Autodesk Inventor part; units mm, degrees
ref_plane "YZ Plane" through (0, 0, 0) normal (1, 0, 0) x (0, 1, 0)
ref_plane "XZ Plane" through (0, 0, 0) normal (0, 1, 0) x (-1, 0, 0)
ref_plane "XY Plane" through (0, 0, 0) normal (0, 0, 1) x (1, 0, 0)
sketch "Sketch1" plane through (0, 0, 0) normal (1, 0, 0) x (0, 1, 0)
  line L0 (0, 0) -> (25.4, 0)
  line L1 (0, 0) -> (0, -25.4)
  line L2 (25.4, -6.35) -> (6.35, -6.35)
  line L3 (6.35, -6.35) -> (6.35, -25.4)
  line L4 (6.35, -25.4) -> (0, -25.4)
  line L5 (25.4, 0) -> (25.4, -6.35)
  dimension "d0" = 25.4
  dimension "d1" = 25.4
  dimension "d2" = 6.35
extrude "Extrusion1" add sketch "Sketch1" along normal mid plane 120
sketch "Sketch2" plane through (-60, 6.35, -6.35) normal (0, 1, 0) x (1, 0, 0)
  circle A0 centre (10, 9.525) radius 4.1
  line L0 (0, 0) -> (0, 19.05) construction
  line L1 (0, 19.05) -> (120, 19.05) construction
  circle A1 centre (30, 9.525) radius 4.1
  circle A2 centre (50, 9.525) radius 4.1
  circle A3 centre (70, 9.525) radius 4.1
  circle A4 centre (90, 9.525) radius 4.1
  circle A5 centre (110, 9.525) radius 4.1
  point P0 (60, -6.35)
  point P1 (0, 9.525)
  point P2 (0, 9.525)
  dimension "d5" = 8.2
  dimension "d6" = 10
  dimension "d9" = 20
hole "Hole1" at (50, 6.35, -15.875) at (30, 6.35, -15.875) at (10, 6.35, -15.875) at (-10, 6.35, -15.875) at (-30, 6.35, -15.875) at (-50, 6.35, -15.875) direction (0, -1, 0) diameter 8.2 end through all countersink diameter 14 countersink angle 90
sketch "Sketch3" plane through (60, 25.4, -6.35) normal (0, 0, -1) x (-1, 0, 0)
  circle A0 centre (10, -9.525) radius 4
  line L0 (0, -19.05) -> (0, 0) construction
  line L1 (120, 0) -> (0, 0) construction
  circle A1 centre (30, -9.525) radius 4
  circle A2 centre (50, -9.525) radius 4
  circle A3 centre (70, -9.525) radius 4
  circle A4 centre (90, -9.525) radius 4
  circle A5 centre (110, -9.525) radius 4
  point P0 (60, -25.4)
  point P1 (0, -9.525)
  dimension "d21" = 8
  dimension "d22" = 10
  dimension "d25" = 20
hole "Hole2" at (50, 15.875, -6.35) at (30, 15.875, -6.35) at (10, 15.875, -6.35) at (-10, 15.875, -6.35) at (-30, 15.875, -6.35) at (-50, 15.875, -6.35) direction (0, 0, 1) diameter 8.2 end through all countersink diameter 14 countersink angle 90
properties part number "MotorMountingBracket"
Source: CAD feature listing. Evaluate the final solid. Frame: model axes, mm. A direction names the side the tool comes from. Coordinates: 2 decimals unless noted, no trailing zeros. Order: outer loops, then holes, each group sorted by start corner. A loop starts at its lowest first (then second) coordinate and runs counter-clockwise, first axis right, second up. Notation, with made-up numbers: M -13.5,16 L -0.5,16 A10 cw -0.5,30 Z; hole C 85.5,1 d8. An arc over 180 degrees is marked long. Write each question's results on one line, items separated by ' | '. Start each with the question number.
1) Section query A-A (x = 10). Return the cut outline in (y, z) (3 decimals), plus the area to 3 significant figures.
2) Contact query for flat-ended pins moving along their axis: pin 1 Ø13 at (x, z) = (30, -15.875) entering from +Y; pin 2 Ø13 at (x, y) = (-30, 15.875) entering from -Z; pin 3 Ø2 at (x, y) = (28.5, 11.5) entering from -Z (3 decimals); pin 4 Ø8 at (x, z) = (-16.5, -17) entering from -Y. Output: stop coordinate, or through.
3) Draft query along Z for faces 1 (the face through (-32.61, 3.63, -19.27)), 2 (the face through (7.39, 12.48, -3.63)), 3 (the face through (-1, 0, -13)). Return one class per face: released by +Z, released by -Z, zero draft, split by the parting line, or undercut.
4) Access query for faces 4 (the face through (-1, 16, -6.35)), 5 (the face through (-27.51, 1.7, -19.13)). Directions: +Z, -Z, +X, -X, +Y, -Y. A direction counts if a zero-diameter tool reaches every point of the face in a straight line with its end or side. Return the directions, or none.
5) Section query B-B (z = -18.75). Give the number of separate pieces and of enclosed holes in the cut face, plus the area to 3 significant figures.
6) Line query: line 1 (Z direction, x = 50, y = 0.75) (3 decimals); line 2 (Z direction, x = -18, y = 19); line 3 (Y direction, x = -24, z = -11). Output: solid intervals per line, ascending. Write a range as from..to.
Answers:
1) outline: M 0,-25.4 L 6.35,-25.4 L 6.35,-22.875 L 3.45,-19.975 L 0,-19.975 Z; M 0,-11.775 L 3.45,-11.775 L 6.35,-8.875 L 6.35,-6.35 L 8.875,-6.35 L 11.775,-3.45 L 11.775,0 L 0,0 Z; M 19.975,-3.45 L 22.875,-6.35 L 25.4,-6.35 L 25.4,0 L 19.975,0 Z | area: 161 mm^2
2) pin 1: stops at y = 5.85 | pin 2: stops at z = -5.85 | pin 3: stops at z = -4.975 | pin 4: stops at y = 0
3) face 1: undercut | face 2: released by -Z | face 3: zero draft
4) face 4: -Z, +X, -X, +Y | face 5: +Y, -Y
5) separate pieces: 7 | enclosed holes: 0 | area: 477 mm^2
6) line 1: z = -25.4..-19.975, -11.775..0 | line 2: z = -6.35..0 | line 3: y = 0..6.35
